Geometry: final body of the model. Coordinates: model frame, mm. A direction names the side the tool comes from. Give positions to 0.01 mm unless a question says otherwise; leave off trailing zeros. Order: outer loops, then holes, each group sorted by start corner. A loop starts at its lowest first (then second) coordinate and runs counter-clockwise, first axis right, second up. Notation, with made-up numbers: (76.25, -10) - (114.25, -10) arc R6 ccw to (114.25, -3) - close; hole circle Ø10 at (88, 83.5). An arc over 180 degrees is marked (long way). Put each result on its own line as item: value. Start each with the question number.
1. Ray query, line 1 along Y through (x, z) = (0.85, 0) (3 decimals); line 2 along X through (y, z) = (3.5, 4.75); line 3 along Y through (x, z) = (-0.9, 0) (3 decimals). Return the intervals inside material, ascending. Write a range as from..to.
2. Section D-D on y = -4.75. Return the cut outline in (x, z).
3. Section B-B on z = 0. Return the cut outline in (x, y) (3 decimals).
4. Mould query, pull axis Y, two halves, no side actions, for faces 1 (the cylindrical face through (1.77, -4.88, 1.08)), 2 (the flat face through (-1.5, -4, 0)), 3 (the flat face through (-1, 0.75, -5)). Classes: pulls with the +Y half, pulls with the -Y half, needs draft (parallel to the pull), parting line crosses it, or undercut.
5. Set-up query: faces 4 (the flat face through (-1, -0.75, -5)), 5 (the flat face through (0, 4, 4)), 6 (the flat face through (-1.5, 4, 0)). Return all of +Z, -Z, +X, -X, +Y, -Y with unobstructed straight access to the full face (end or side cutting, diameter ignored); none if empty.
6. First-contact query: P1, Ø0.8, axis at x = -1, z = -4.5, coming from the -Y side; P2, Ø0.5, axis at x = -1, z = 4.5, coming from the +Y side; P3, Ø3, axis at x = 2, y = 4, coming from the -Z side; P4, Ø3.5, axis at y = 1, z = 0.5, coming from the +X side. Flat tips, straight axial feed; report the tip coordinate or a pass-through.
7. Section C-C on x = 1.25. Return the cut outline in (y, z) (3 decimals).
8. Section A-A on y = 0. Return the cut outline in (x, z) (3 decimals), plus the area to 3 significant figures.
from build123d import *

# Parameters (mm, degrees)
ESQUISSE1_R                  = 5
ESQUISSE1_R_2                = 3.375
EXTRUSION1_DEPTH             = 3.5
EXTRUSION1_DEPTH_BACK        = 1.5
ESQUISSE2_R                  = 6
ESQUISSE2_R_2                = 3.375
EXTRUSION2_DEPTH             = 1.5
ESQUISSE3_W                  = 1
ESQUISSE3_H                  = 1.5
ENL_V_MAT_EXTRU_1_DEPTH      = 7
ENL_V_MAT_EXTRU_1_DEPTH_BACK = 7


with BuildPart() as part:
    # Esquisse1 → Extrusion1 (new body, two sides)
    with BuildSketch(Plane(origin=(0, 0, 0), x_dir=(0, 0, -1), z_dir=(1, 0, 0))) as extrusion1_sk:
        Circle(ESQUISSE1_R)
        Circle(ESQUISSE1_R_2, mode=Mode.SUBTRACT)
    extrude(amount=EXTRUSION1_DEPTH)
    extrude(extrusion1_sk.sketch, amount=-EXTRUSION1_DEPTH_BACK)

    # Esquisse2 → Extrusion2 (add)
    with BuildSketch(Plane(origin=(0, 0, 0), x_dir=(0, 0, -1), z_dir=(1, 0, 0))):
        Circle(ESQUISSE2_R)
        Circle(ESQUISSE2_R_2, mode=Mode.SUBTRACT)
    extrude(amount=-EXTRUSION2_DEPTH)

    # Esquisse3 → Enlèv. mat.-Extru.1 (cut, two sides)
    with BuildSketch(Plane.XY) as enl_v_mat_extru_1_sk:
        with Locations((-1, 0)):
            Rectangle(ESQUISSE3_W, ESQUISSE3_H)
    extrude(amount=ENL_V_MAT_EXTRU_1_DEPTH, mode=Mode.SUBTRACT)
    extrude(enl_v_mat_extru_1_sk.sketch, amount=-ENL_V_MAT_EXTRU_1_DEPTH_BACK, mode=Mode.SUBTRACT)


solid = part.part
Resolved:
1. line 1: -5..-3.375, 3.375..5
1. line 2: -1.5..0
1. line 3: -6..-3.375, 3.375..6
2. outline: (-1.5, -3.67) - (0, -3.67) - (0, -1.56) - (3.5, -1.56) - (3.5, 1.56) - (0, 1.56) - (0, 3.67) - (-1.5, 3.67) - close
3. outline: (-1.5, -6) - (0, -6) - (0, -5) - (3.5, -5) - (3.5, -3.375) - (-1.5, -3.375) - close; (-1.5, 3.375) - (3.5, 3.375) - (3.5, 5) - (0, 5) - (0, 6) - (-1.5, 6) - close
4. face 1: parting line crosses it
4. face 2: needs draft
4. face 3: undercut
5. face 4: +Z, -Z, -X
5. face 5: +X
5. face 6: +Z, -Z, -X, +Y, -Y
6. P1: y = -4.38
6. P2: y = 4.24
6. P3: z = -4.33
6. P4: through
7. outline: circle Ø10 at (0, 0); hole circle Ø6.75 at (0, 0)
8. outline: (-0.5, -6) - (0, -6) - (0, -5) - (3.5, -5) - (3.5, -3.375) - (-0.5, -3.375) - close; (-0.5, 3.375) - (3.5, 3.375) - (3.5, 5) - (0, 5) - (0, 6) - (-0.5, 6) - close
8. area: 14.0 mm^2
